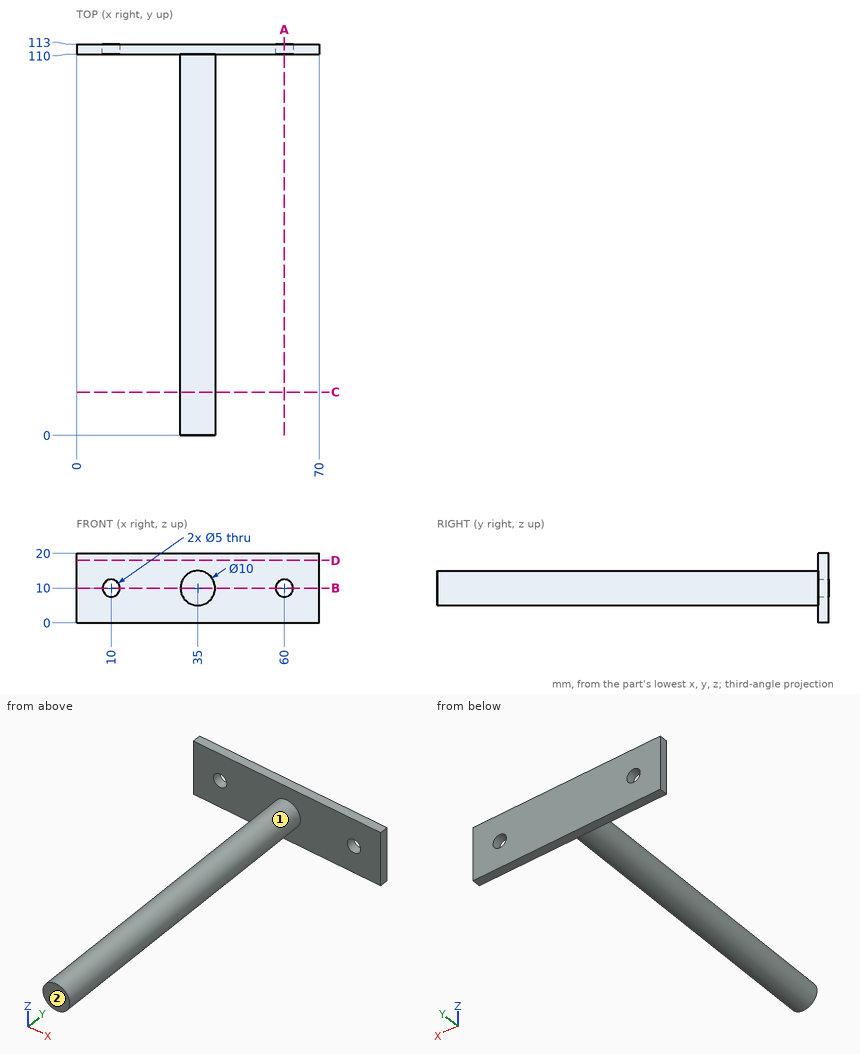
Geometry: see drawing. Coordinates: mm, zero at the bounding-box minimum. A direction names the side the tool comes from. Give positions to 0.01 mm unless a question says otherwise; leave off trailing zeros. Order: outer loops, then holes, each group sorted by start corner. A loop starts at its lowest first (then second) coordinate and runs counter-clockwise, first axis right, second up. Notation, with made-up numbers: (57, -1) - (73, -1) arc R31 ccw to (73, 27) - close; hole circle Ø5 at (-30, -8.5). An arc over 180 degrees is marked (long way). Use CSV: the item, a comma, the result in double quotes.
1. Section query A-A (x = 60). Output: boundary loops of the cut face in (y, z), plus the area to 3 significant figures.
Answers below:
outline,"(110, 0) - (113, 0) - (113, 7.5) - (110, 7.5) - close; (110, 12.5) - (113, 12.5) - (113, 20) - (110, 20) - close"
area,"45.0 mm2"
2. Section query C-C (y = 12.5). Output: boundary loops of the cut face in (x, z).
Answers below:
outline,"circle Ø10 at (35, 10)"
3. Section query B-B (z = 10). Output: boundary loops of the cut face in (x, y), plus the area to 3 significant figures.
Answers below:
outline,"(0, 110) - (7.5, 110) - (7.5, 113) - (0, 113) - close; (12.5, 110) - (30, 110) - (30, 0) - (40, 0) - (40, 110) - (57.5, 110) - (57.5, 113) - (12.5, 113) - close; (62.5, 110) - (70, 110) - (70, 113) - (62.5, 113) - close"
area,"1,280 mm2"
4. Section query D-D (z = 18). Output: boundary loops of the cut face in (x, y), plus the area to 3 significant figures.
Answers below:
outline,"(0, 110) - (70, 110) - (70, 113) - (0, 113) - close"
area,"210 mm2"
5. Material intervals for line 1 along Z through (x, y) = (60, 111); line 2 along Y through (x, z) = (27, 17); line 3 along X through (y, z) = (74, 9), sorted ascending. Write a range as from..to.
Answers below:
line 1,"0..7.5, 12.5..20"
line 2,"110..113"
line 3,"30.1..39.9"
6. Contact query for flat-ended pins moving along their axis: pin 1 (1.5 mm diameter, centred on x = 50.5, z = 4.5, fed in from -Y); pin 2 (3 mm diameter, centred on y = 36, z = 14.5, fed in from -X); pin 3 (12 mm diameter, centred on x = 25, y = 76, fed in from +Z). Output: stop coordinate, or through.
Answers below:
pin 1,"y = 110"
pin 2,"x = 31"
pin 3,"z = 13"
7. Access query for the marked faces 1 and 2. Directions: +Z, -Z, +X, -X, +Y, -Y. A direction counts if a zero-diameter tool reaches every point of the face in a straight line with its end or side. Return the directions, or none.
Answers below:
face 1,"-Y"
face 2,"+Z, -Z, +X, -X, -Y"
